For this review, use the dimensioned drawing (mm, ordinates from the lowest corner) and the shaded views. A direction names the side the tool comes from. Coordinates: 2 decimals unless noted, no trailing zeros. Loops run counter-clockwise (first coordinate to the right, second up) from the corner with the lowest first, then second, coordinate; pieces in that order, holes last. Notation, with made-up numbers: M 34.25,73 L 67.25,73 A29 ccw 67.25,108 Z; hole C 81.25,40.25 d7. An arc over 180 degrees is marked long. Write item = value, one per line. Start each with the question number.
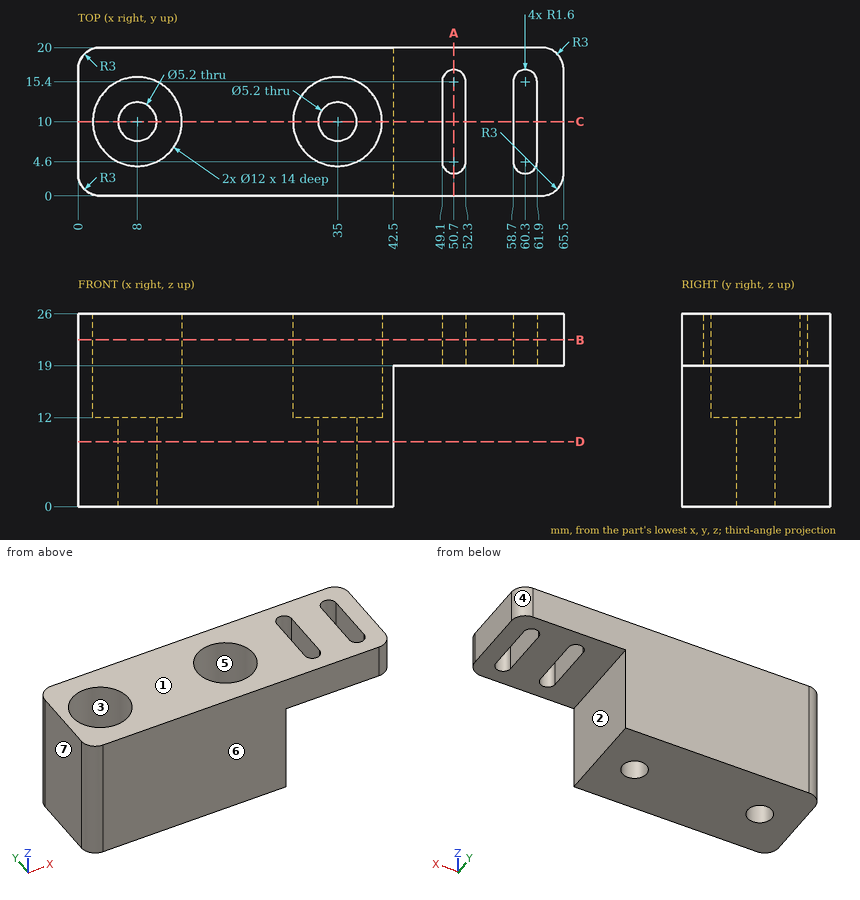
Q1. Add section B-B on z = 22.5. State the section outline as (x, y) points, plus the area to 3 significant figures.
Q2. To check wall thickness, follow line 1 (Y direction, x = 35, z = 23.25); line 2 (X direction, y = 8, z = 21); line 3 (X direction, y = 9.5, z = 23.75). State the ranges of each line that lie inside material, in increasing order. Write a range as from..to.
Q3. Add section C-C on y = 10. Give the number of separate pieces and of enclosed holes in the cut face, plus the area to 3 significant figures.
Q4. For the marked faces 1, 2 and 3, list the 3-axis set-ups (+Z, -Z, +X, -X, +Y, -Y) from which the entire face can be reached by the end or side of a thin tool; tool diameter is ignored.
Q5. Add section D-D on z = 8.75. State the section outline as (x, y) points, plus the area to 3 significant figures.
Q6. Clearance check with flat-ended pins moving along their axes: P1, Ø10, axis at y = 16.5, z = 17, coming from the +X side; P2, Ø6, axis at y = 10, z = 9, coming from the +X side; P3, Ø6, axis at x = 49, y = 12, coming from the -Z side. State where each tip first meets the part, or that it passes through.
Q7. Mouldability with a two-part tool opening along X and no side actions: class the marked faces 4, 5, 6 and 7 as released by +X, released by -X, zero draft, split by the parting line, or undercut.
Q8. Add section A-A on x = 50.7. State the section outline as (y, z) points, plus the area to 3 significant figures.
Values follow:
q1.outline = M 0,3 A3 ccw 3,0 L 62.5,0 A3 ccw 65.5,3 L 65.5,17 A3 ccw 62.5,20 L 3,20 A3 ccw 0,17 Z; hole C 8,10 d12; hole C 35,10 d12; hole M 49.1,4.6 A1.6 ccw 52.3,4.6 L 52.3,15.4 A1.6 ccw 49.1,15.4 Z; hole M 58.7,4.6 A1.6 ccw 61.9,4.6 L 61.9,15.4 A1.6 ccw 58.7,15.4 Z
q1.area = 991 mm2
q2.line_1 = 0..4, 16..20
q2.line_2 = 0..2.34, 13.66..29.34, 40.66..49.1, 52.3..58.7, 61.9..65.5
q2.line_3 = 0..2.02, 13.98..29.02, 40.98..49.1, 52.3..58.7, 61.9..65.5
q3.separate_pieces = 5
q3.enclosed_holes = 0
q3.area = 760 mm2
q4.face_1 = +Z, +X, -X, +Y, -Y
q4.face_2 = -Z, +X, +Y, -Y
q4.face_3 = +Z
q5.outline = M 0,3 A3 ccw 3,0 L 42.5,0 L 42.5,20 L 3,20 A3 ccw 0,17 Z; hole C 8,10 d5.2; hole C 35,10 d5.2
q5.area = 804 mm2
q6.P1 = 65.5
q6.P2 = 42.5
q6.P3 = 19
q7.face_4 = released by +X
q7.face_5 = undercut
q7.face_6 = zero draft
q7.face_7 = released by -X
q8.outline = M 0,19 L 3,19 L 3,26 L 0,26 Z; M 17,19 L 20,19 L 20,26 L 17,26 Z
q8.area = 42.0 mm2
